Could you check a few things on this drawing? It's one solid part, dimensions in mm from its lowest x, y, z. Give positions to 0.01 mm unless a question says otherwise; leave off trailing zeros. Write each loop counter-clockwise with the first axis right and the second up, starting at its lowest first coordinate (ties: lowest second). Pieces come first, ordered by that corner, then holes. Notation, with made-up numbers: (-7, 54.25) - (42, 54.25) arc R28 cw to (42, 86.25) - close; hole circle Ø10 at (81, 83.5). An arc over 180 degrees is marked (long way). One line per item, written item: value. Start each with the question number.
1) We'd pull the mould along Z, two halves only. Please class the marked faces 1 and 2: +Z half, -Z half, draft (parallel to the pull), parting line (faces both ways), or undercut.
2) Please list where these lines run through material, in increasing order: L1, parallel to Z at x = 43.5, y = 2.65; L2, parallel to Z at x = 19.06, y = 0.35 (1 decimal); L3, parallel to Y at x = 51, z = 31. Write a range as [from, to].
3) Imagine slicing it at D-D on x = 30. Write out the boundary of the cut face in (y, z).
4) Imagine slicing it at B-B on x = 8.9. Write out the boundary of the cut face in (y, z) (1 decimal).
5) I'm going to push flat-ended pins straight in: P1, Ø0.7, axis at y = 1.5, z = 37, coming from the +X side; P2, Ø19, axis at x = 40.5, z = 14.5, coming from the +Y side; P3, Ø0.7, axis at y = 1.5, z = 37, coming from the -X side. Where does each tip first touch, or does it pass through?
6) Imagine slicing it at A-A on y = 1.9. Write out the boundary of the cut face in (x, z).
7) Imagine slicing it at C-C on z = 27.5. Write out the boundary of the cut face in (x, y).
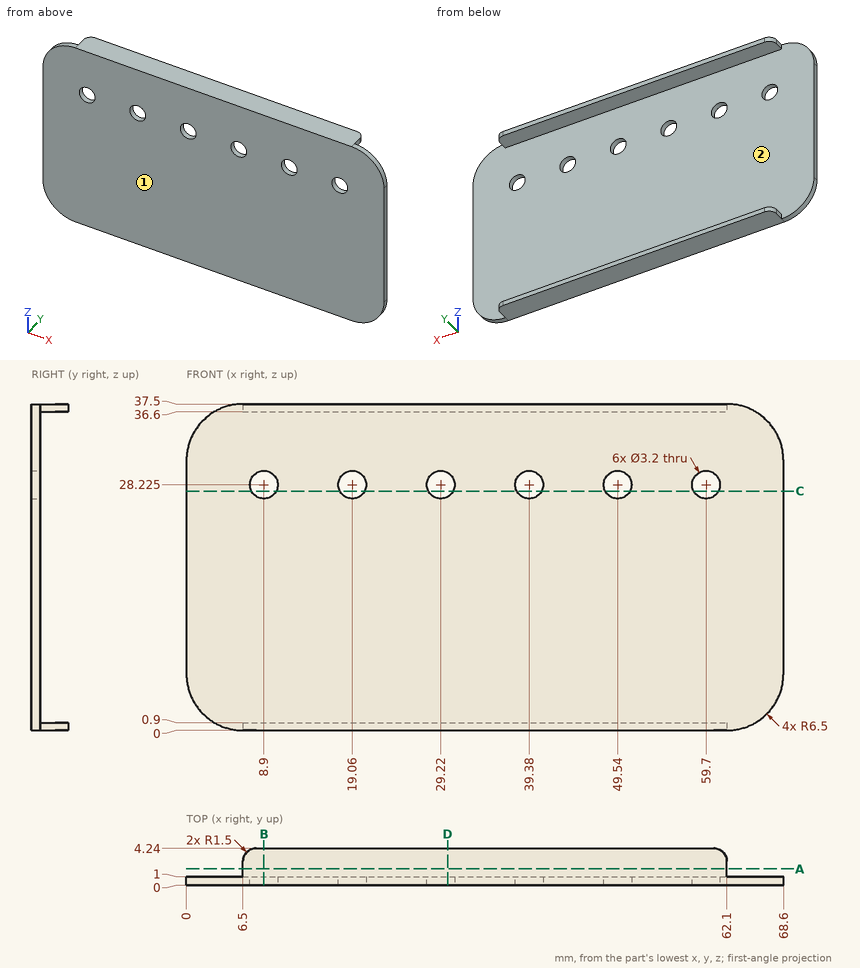
Numbers:
1. face 1: draft
1. face 2: undercut
2. L1: [0, 0.9], [36.6, 37.5]
2. L2: [0, 26.6], [29.8, 37.5]
2. L3: [0, 1]
3. outline: (0, 0) - (4.24, 0) - (4.24, 0.9) - (1, 0.9) - (1, 26.83) - (0, 26.83) - close; (0, 29.62) - (1, 29.62) - (1, 36.6) - (4.24, 36.6) - (4.24, 37.5) - (0, 37.5) - close
4. outline: (0, 0) - (4.2, 0) - (4.2, 0.9) - (1, 0.9) - (1, 26.6) - (0, 26.6) - close; (0, 29.8) - (1, 29.8) - (1, 36.6) - (4.2, 36.6) - (4.2, 37.5) - (0, 37.5) - close
5. P1: x = 62.1
5. P2: y = 1
5. P3: x = 6.5
6. outline: (6.5, 0) - (62.1, 0) - (62.1, 0.9) - (6.5, 0.9) - close; (6.5, 36.6) - (62.1, 36.6) - (62.1, 37.5) - (6.5, 37.5) - close
7. outline: (0, 0) - (7.47, 0) - (7.47, 1) - (0, 1) - close; (10.33, 0) - (17.63, 0) - (17.63, 1) - (10.33, 1) - close; (20.49, 0) - (27.79, 0) - (27.79, 1) - (20.49, 1) - close; (30.65, 0) - (37.95, 0) - (37.95, 1) - (30.65, 1) - close; (40.81, 0) - (48.11, 0) - (48.11, 1) - (40.81, 1) - close; (50.97, 0) - (58.27, 0) - (58.27, 1) - (50.97, 1) - close; (61.13, 0) - (68.6, 0) - (68.6, 1) - (61.13, 1) - close
